Can you work these out from the model? Positions are in its coordinate system, mm. Face numbers are marked on the shaded views. A direction names the side the tool comes from. Give positions to 0.01 mm unless a question says otherwise; leave off trailing zeros. Loops run counter-clockwise (first coordinate to the right, second up) from the corner with the lowest first, then second, coordinate; pieces in that order, holes last. Notation, with made-up numbers: (7.25, 30) -> (47.25, 30) arc R17 ccw to (47.25, 46) -> close; hole circle Ø8 at (-36, 50.5). An arc over 180 degrees is marked (long way). Return JSON: item names as keys, results as strings. Group by question number.
Q1. Suppose I cut it at B-B, the plane z = 2.5. Please give me the cut outline in (x, y) (3 decimals).
Q2. Suppose I cut it at D-D, the plane y = -8. Please give me the cut outline in (x, z), and give its area (3 significant figures).
Q3. Suppose I cut it at A-A, the plane y = 14.5. Please give me the cut outline in (x, z).
Q4. Will these pins go through, and if not, where does the flat tip stop? pin 1 (1.8 mm diameter, centred on x = 0, y = 0, fed in from -Z); pin 2 (1 mm diameter, centred on x = 1.5, z = 4.5, fed in from -Y); pin 3 (3 mm diameter, centred on x = 0, y = -0.5, fed in from +Z); pin 4 (2 mm diameter, centred on x = -4.5, y = -11.5, fed in from -Z).
Q5. Thinking about a two-plate mould opening in Y: for the marked faces 4, 5 and 6, which applies, pulls with the +Y half, pulls with the -Y half, needs draft (parallel to the pull), parting line crosses it, or undercut?
Q6. Suppose I cut it at C-C, the plane x = 5.5. Please give me the cut outline in (y, z), and give its area (3 significant figures).
Q7. Which directions (+Z, -Z, +X, -X, +Y, -Y) give clear straight access to the entire face, cutting with the end or side of a thin tool? Please do the marked faces 1, 2 and 3.
Q8. I need wall thicknesses on line 1 along Y through (x, z) = (0, 5.75) (3 decimals); line 2 along Y through (x, z) = (0, -9.7); line 3 along Z through (x, y) = (-5, -11.5). Which ranges of each line are inside material? Lowest first, please. Write a range as [from, to].
```python
from build123d import *

# Parameters (mm, degrees)
F0_R      = 19
F1_DEPTH  = 7
F2_R      = 11.25
F3_DEPTH  = 2
F4_R      = 14
F4_R_2    = 6.4
F5_DEPTH  = 3
F8_DEPTH  = 6
F9_R      = 1.5
F10_DEPTH = 12


# Not quite as in the source:
# - a feature names something its author has since deleted; it is built from what else it names


with BuildPart() as f1:
    # F0 (on Top) → F1 (new body)
    with BuildSketch(Plane.XY):
        Circle(F0_R)
    extrude(amount=F1_DEPTH)

    # F2 (on face) → F3 (join)
    with BuildSketch(Plane(origin=(0, 0, 0), x_dir=(1, 0, 0), z_dir=(0, 0, -1))):
        Circle(F2_R)
    extrude(amount=F3_DEPTH)

    # F4 (on face) → F5 (cut)
    with BuildSketch(Plane.XY.offset(7)):
        Circle(F4_R)
        Circle(F4_R_2, mode=Mode.SUBTRACT)
    extrude(amount=-F5_DEPTH, mode=Mode.SUBTRACT)

    # F6: F1 across face


with BuildPart() as f1_1:
    add(f1.part)
    add(f1.part.mirror(Plane(origin=(0, 0, -2), x_dir=(1, 0, 0), z_dir=(0, 0, -1))))

    # F7 (on face) → F8 (cut)
    with BuildSketch(Plane.XY.offset(7)):
        with BuildLine():
            Line((1.942775077, 1.875), (-1.942775077, 1.875))
            ThreePointArc((-1.942775077, 1.875), (-2.7, 0), (-1.942775077, -1.875))
            Line((-1.942775077, -1.875), (1.942775077, -1.875))
            ThreePointArc((1.942775077, -1.875), (2.7, 0), (1.942775077, 1.875))
        make_face()
    extrude(amount=-F8_DEPTH, mode=Mode.SUBTRACT)

    # F9 (on face) → F10 (cut, through all)
    with BuildSketch(Plane(origin=(0, 0, -11), x_dir=(1, 0, 0), z_dir=(0, 0, -1))):
        Circle(F9_R)
    extrude(amount=-F10_DEPTH, mode=Mode.SUBTRACT)


solid = f1_1.part
```
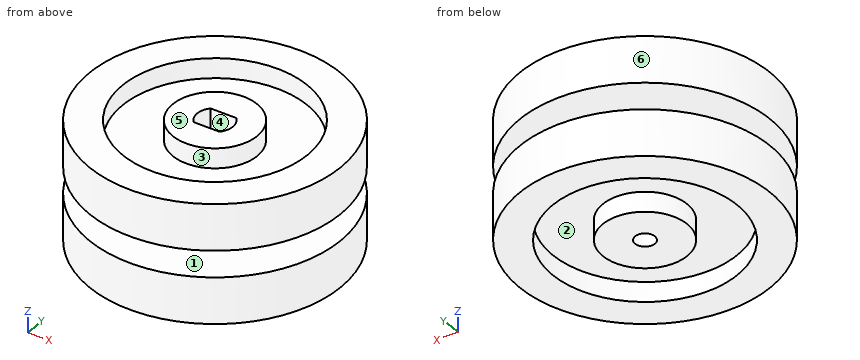
Ans:
{
 "1": {"outline": "circle Ø38 at (0, 0); hole (-1.943, -1.875) -> (1.943, -1.875) arc R2.7 ccw to (1.943, 1.875) -> (-1.943, 1.875) arc R2.7 ccw to start"},
 "2": {"outline": "(-17.23, -11) -> (-11.49, -11) -> (-11.49, -8) -> (11.49, -8) -> (11.49, -11) -> (17.23, -11) -> (17.23, -4) -> (7.91, -4) -> (7.91, 0) -> (17.23, 0) -> (17.23, 7) -> (11.49, 7) -> (11.49, 4) -> (-11.49, 4) -> (-11.49, 7) -> (-17.23, 7) -> (-17.23, 0) -> (-7.91, 0) -> (-7.91, -4) -> (-17.23, -4) -> close", "area": "408 mm^2"},
 "3": {"outline": "(-12.28, -11) -> (12.28, -11) -> (12.28, -4) -> (-12.28, -4) -> close; (-12.28, 0) -> (12.28, 0) -> (12.28, 7) -> (-12.28, 7) -> close"},
 "4": {"pin 1": "passes through", "pin 2": "stops at y = -18.97", "pin 3": "stops at z = 7", "pin 4": "stops at z = -8"},
 "5": {"face 4": "undercut", "face 5": "needs draft", "face 6": "parting line crosses it"},
 "6": {"outline": "(-18.19, -11) -> (-12.87, -11) -> (-12.87, -8) -> (-3.27, -8) -> (-3.27, -11) -> (3.27, -11) -> (3.27, -8) -> (12.87, -8) -> (12.87, -11) -> (18.19, -11) -> (18.19, -4) -> (9.81, -4) -> (9.81, 0) -> (18.19, 0) -> (18.19, 7) -> (12.87, 7) -> (12.87, 4) -> (3.27, 4) -> (3.27, 7) -> (-3.27, 7) -> (-3.27, 4) -> (-12.87, 4) -> (-12.87, 7) -> (-18.19, 7) -> (-18.19, 0) -> (-9.81, 0) -> (-9.81, -4) -> (-18.19, -4) -> close", "area": "473 mm^2"},
 "7": {"face 1": "none", "face 2": "-Z", "face 3": "+Z"},
 "8": {"line 1": "y = [-19, -14], [-6.4, -1.875], [1.875, 6.4], [14, 19]", "line 2": "y = [-19, -14], [-6.4, -1.5], [1.5, 6.4], [14, 19]", "line 3": "z = [-8, -4], [0, 4]"}
}
